Can you work these out from the drawing? Everything is in mm from the part's minimum corner. A direction names the side the tool comes from. Round coordinates to 2 decimals unless told otherwise and drop trailing zeros. Order: outer loops, then holes, each group sorted by start corner. A loop starts at its lowest first (then second) coordinate and runs counter-clockwise, first axis right, second up. Notation, with made-up numbers: (38, 87.25) -> (89, 87.25) arc R18 ccw to (89, 121.25) -> close; hole circle Ø10 at (24.5, 35.25). An arc over 180 degrees is marked (long way). Use a Markdown table: item, result. Add a question column.
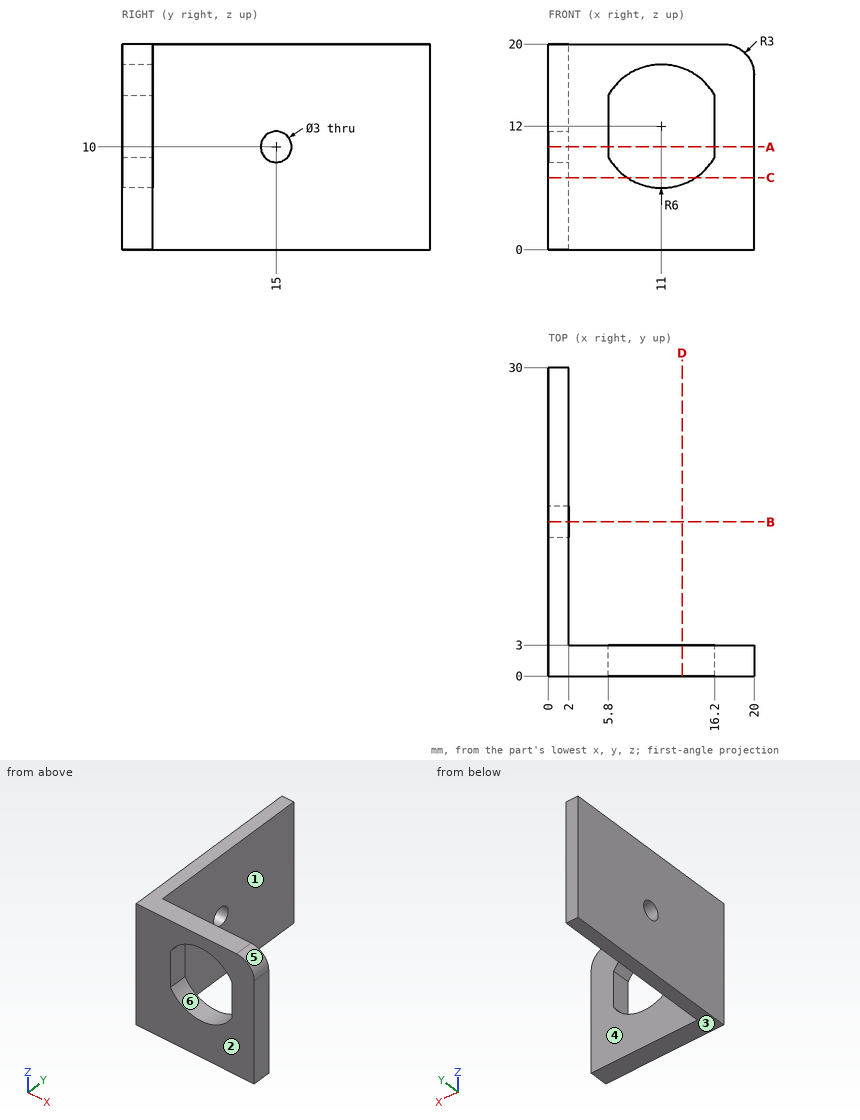
(1) I want a section at D-D on x = 13. List the corners of the cut face in (y, z) for me, and give its area (3 significant figures).
(2) If we mould it in two halves opening along Z, with no side actions, what happens to the marked faces 3, 4, 5 and 6? For each: pulls with the +Z half, pulls with the -Z half, needs draft (parallel to the pull), parting line crosses it, or undercut.
(3) On a 3-axis mill with a long thin cutter (end or side, diameter ignored), from which of +Z, -Z, +X, -X, +Y, -Y can I reach the whole of each face in a straight line? I mean the marked faces 1 and 2. Say none if no direction works.
(4) I want a section at B-B on y = 15. List the corners of the cut face in (x, z) for me.
(5) Please list where these lines run through material, in increasing order: probe 1 along Z at (x, y) = (1.25, 15); probe 2 along Y at (x, z) = (5.5, 2.75); probe 3 along X at (y, z) = (21, 11.75). Write a range as from..to.
(6) I want a section at A-A on z = 10. List the corners of the cut face in (x, y) for me.
(7) I want a section at C-C on z = 7. List the corners of the cut face in (x, y) for me.
(8) I'm going to push flat-ended pins straight in: P1, Ø3, axis at y = 20.5, z = 5, coming from the +X side; P2, Ø12, axis at x = 10, y = 25.5, coming from the +Z side; P3, Ø1.5, axis at x = 2.5, y = 10, coming from the -Z side; P4, Ø9, axis at x = 14.5, z = 9, coming from the +Y side. Where does each tip first touch, or does it pass through?
Output:
| question | item | result |
|---|---|---|
| 1 | outline | (0, 0) -> (3, 0) -> (3, 6.34) -> (0, 6.34) -> close; (0, 17.66) -> (3, 17.66) -> (3, 20) -> (0, 20) -> close |
| 1 | area | 26.1 mm² |
| 2 | face 3 | pulls with the -Z half |
| 2 | face 4 | needs draft |
| 2 | face 5 | pulls with the +Z half |
| 2 | face 6 | undercut |
| 3 | face 1 | +Z, -Z, +X, +Y |
| 3 | face 2 | +Z, -Z, +X, -X, -Y |
| 4 | outline | (0, 0) -> (2, 0) -> (2, 8.5) -> (0, 8.5) -> close; (0, 11.5) -> (2, 11.5) -> (2, 20) -> (0, 20) -> close |
| 5 | probe 1 | 0..8.5, 11.5..20 |
| 5 | probe 2 | 0..3 |
| 5 | probe 3 | 0..2 |
| 6 | outline | (0, 0) -> (5.8, 0) -> (5.8, 3) -> (2, 3) -> (2, 13.5) -> (0, 13.5) -> close; (0, 16.5) -> (2, 16.5) -> (2, 30) -> (0, 30) -> close; (16.2, 0) -> (20, 0) -> (20, 3) -> (16.2, 3) -> close |
| 7 | outline | (0, 0) -> (7.68, 0) -> (7.68, 3) -> (2, 3) -> (2, 30) -> (0, 30) -> close; (14.32, 0) -> (20, 0) -> (20, 3) -> (14.32, 3) -> close |
| 8 | P1 | x = 2 |
| 8 | P2 | through |
| 8 | P3 | z = 0 |
| 8 | P4 | y = 3 |
